Here's the drawing with two shaded views (mm, measured from the low corner). I have some questions. A direction names the side the tool comes from. Give positions to 0.01 mm unless a question says otherwise; leave off trailing zeros. Write each loop counter-clockwise with the first axis right and the second up, starting at its lowest first coordinate (ties: lowest second). Pieces come first, ordered by that corner, then holes.
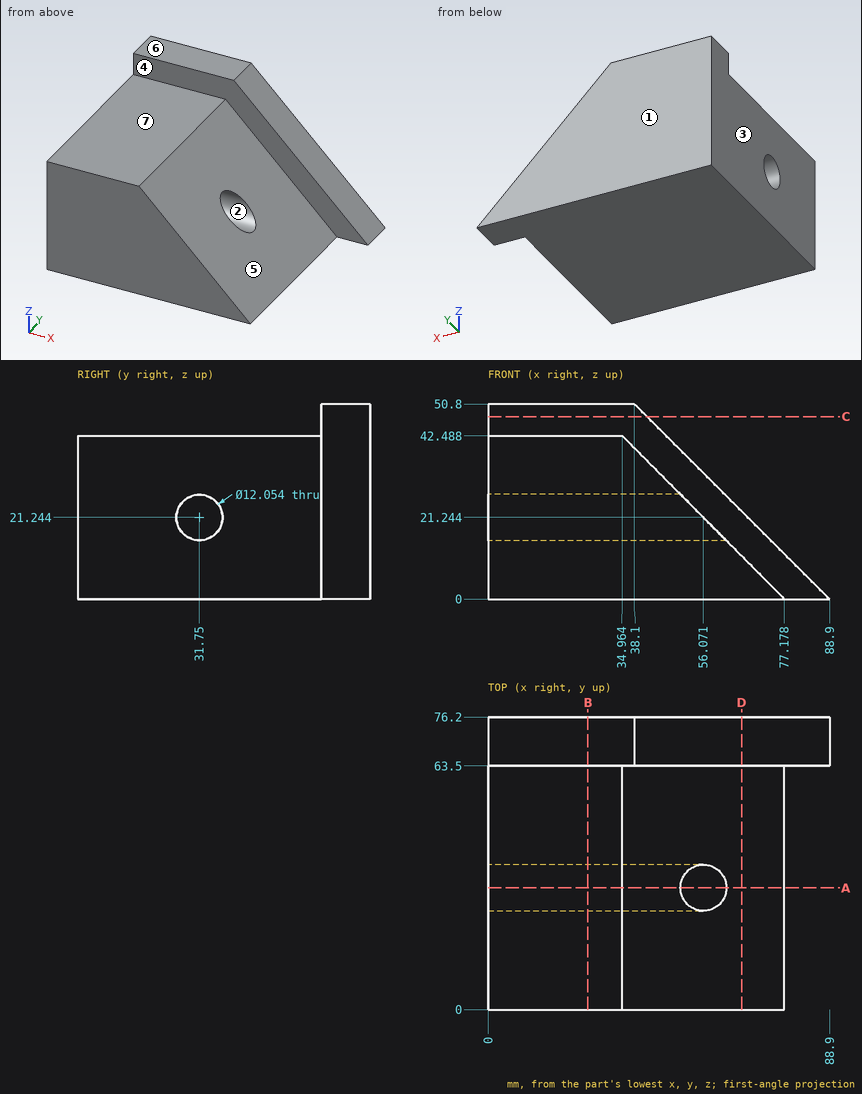
(1) If I drill on L1, parallel to Z at x = 25.5, y = 31.75; L2, parallel to Z at x = 25.5, y = 14; L3, parallel to Z at x = 48, y = 31 (1 decimal), over which ranges is the centre line in solid material (lowest first)?
Returned:
L1: z = 0 to 15.22, 27.27 to 42.49
L2: z = 0 to 42.49
L3: z = 0 to 15.3, 27.2 to 29.4
(2) Imagine slicing it at C-C, the plane z = 47.5. Write out the boundary of the cut face in (x, y), plus the area to 3 significant figures.
Returned:
outline: (0, 63.5) - (41.4, 63.5) - (41.4, 76.2) - (0, 76.2) - close
area: 526 mm2
(3) If we mould it in two halves opening along Y, with no side actions, what happens to the marked faces 1, 2, 3 and 4? For each: +Y half, -Y half, draft (parallel to the pull), parting line (faces both ways), or undercut.
Returned:
face 1: +Y half
face 2: undercut
face 3: draft
face 4: -Y half
(4) Imagine slicing it at A-A, the plane y = 31.75. Write out the boundary of the cut face in (x, z), plus the area to 3 significant figures.
Returned:
outline: (0, 0) - (77.18, 0) - (62.06, 15.22) - (0, 15.22) - close; (0, 27.27) - (50.08, 27.27) - (34.96, 42.49) - (0, 42.49) - close
area: 1,710 mm2
(5) Will these pins go through, and if not, where does the flat tip stop? P1, Ø7, axis at y = 31.75, z = 21.24, coming from the -X side; P2, Ø4, axis at x = 51.5, y = 49.5, coming from the +Z side; P3, Ø1, axis at y = 8.5, z = 14.5, coming from the +X side.
Returned:
P1: passes through
P2: stops at z = 27.86
P3: stops at x = 63.27
(6) Imagine slicing it at B-B, the plane x = 26. Write out the boundary of the cut face in (y, z).
Returned:
outline: (0, 0) - (76.2, 0) - (76.2, 50.8) - (63.5, 50.8) - (63.5, 42.49) - (0, 42.49) - close; hole circle Ø12.05 at (31.75, 21.24)
(7) Imagine slicing it at D-D, the plane x = 66. Write out the boundary of the cut face in (y, z), plus the area to 3 significant figures.
Returned:
outline: (0, 0) - (76.2, 0) - (76.2, 22.9) - (63.5, 22.9) - (63.5, 11.25) - (0, 11.25) - close
area: 1,010 mm2
(8) For the marked faces 5, 6 and 7, which set-ups out of +Z, -Z, +X, -X, +Y, -Y let a thin tool reach every point of the face, with its end or its side?
Returned:
face 5: +Z, +X, -Y
face 6: +Z, +X, -X, +Y, -Y
face 7: +Z, +X, -X, -Y
